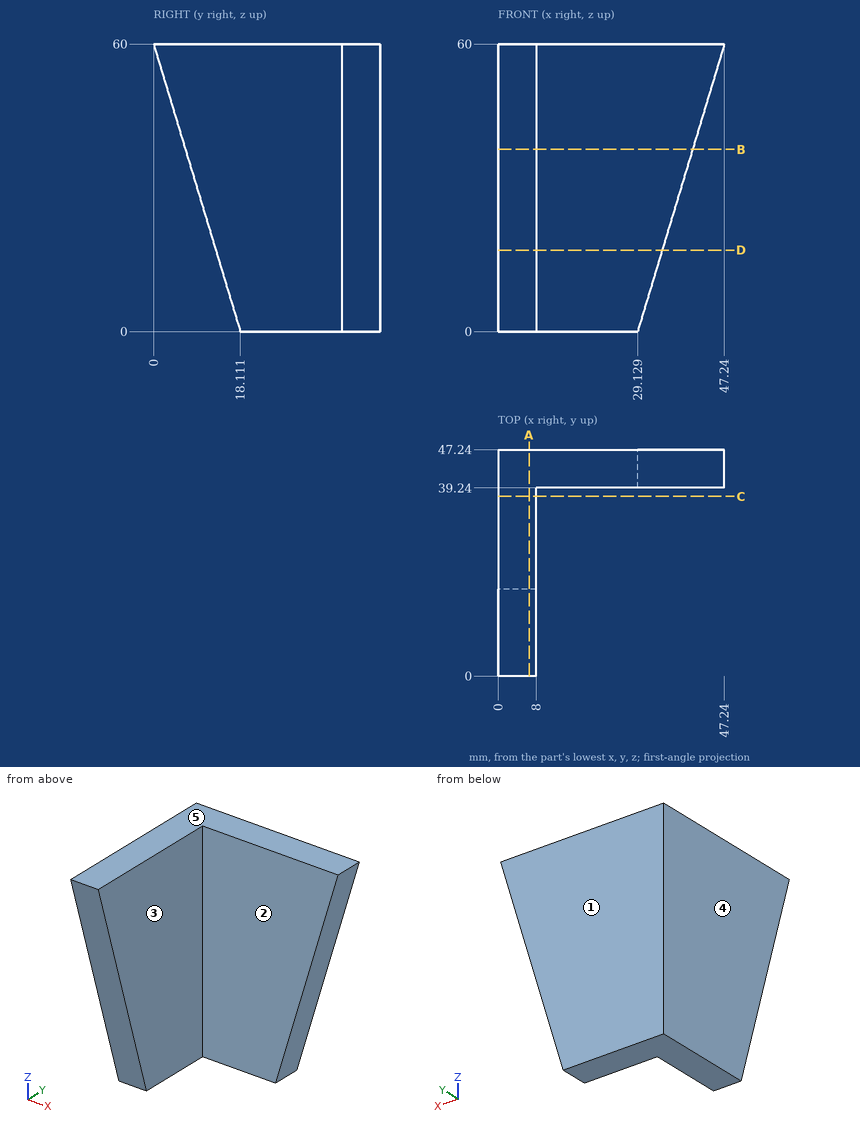
Geometry check sheet. Reference: drawing and pictorial views, mm from the part's lowest x, y, z. A direction names the side the tool comes from. Give positions to 0.01 mm unless a question says otherwise; leave off trailing zeros. Order: outer loops, then holes, each group sorted by start corner. A loop starts at its lowest first (then second) coordinate and runs counter-clockwise, first axis right, second up. Notation, with made-up numbers: M -13.5,-11 L 9.5,-11 A25 ccw 9.5,18 Z; hole C 51.5,85 d5. An arc over 180 degrees is marked long. Answer in a Markdown table with one row per item. Add a question column.
Q1. Sectioned sample at C-C, the plane y = 37.5. Record the boundary of the cut face in (x, z), and give its area (3 significant figures).
Q2. Access from +Z, -Z, +X, -X, +Y, -Y to the whole of each face (thin tool, end or side, straight path). Record for the marked faces 1 and 2.
Q3. Release check for a two-part mould opening along X. For the marked faces 3, 4 and 5 record: released by +X, released by -X, zero draft, split by the parting line, or undercut.
Q4. Thickness scan on L1, parallel to X at y = 7.5, z = 51.5; L2, parallel to Y at x = 12.5, z = 54.5; L3, parallel to Y at x = 2, z = 18.5. Record the ranges inside material, lowest first.
Q5. Sectioned sample at A-A, the plane x = 6.5. Record the boundary of the cut face in (y, z), and give its area (3 significant figures).
Q6. Gauge pin test, flat ends, axial feed: pin 1 Ø8 at (x, z) = (17.5, 31.5) entering from -Y; pin 2 Ø5 at (x, z) = (9, 27) entering from -Y. Record the tip position at first contact, or that the pin passes through.
Q7. Sectioned sample at B-B, the plane z = 38. Record the boundary of the cut face in (x, y).
Q8. Sectioned sample at D-D, the plane z = 17. Record the boundary of the cut face in (x, y).
Verdict:
| question | item | result |
|---|---|---|
| 1 | outline | M 0,0 L 8,0 L 8,60 L 0,60 Z |
| 1 | area | 480 mm² |
| 2 | face 1 | +Z, -Z, +X, -X, +Y |
| 2 | face 2 | +Z, -Z, +X, -Y |
| 3 | face 3 | released by +X |
| 3 | face 4 | released by -X |
| 3 | face 5 | zero draft |
| 4 | L1 | 0 to 8 |
| 4 | L2 | 39.24 to 47.24 |
| 4 | L3 | 12.53 to 47.24 |
| 5 | outline | M 0,60 L 18.11,0 L 47.24,0 L 47.24,60 Z |
| 5 | area | 2,290 mm² |
| 6 | pin 1 | y = 39.24 |
| 6 | pin 2 | y = 9.27 |
| 7 | outline | M 0,6.64 L 8,6.64 L 8,39.24 L 40.6,39.24 L 40.6,47.24 L 0,47.24 Z |
| 8 | outline | M 0,12.98 L 8,12.98 L 8,39.24 L 34.26,39.24 L 34.26,47.24 L 0,47.24 Z |
